```python
from build123d import *

# Parameters (mm, degrees)
CROQUIS1_R              = 1.2
SALIENTE_EXTRUIR1_DEPTH = 1.6
CROQUIS2_W              = 15.7
CROQUIS2_H              = 12.8
SALIENTE_EXTRUIR2_DEPTH = 16


with BuildPart() as part:
    # Croquis1 → Saliente-Extruir1 (new body)
    with BuildSketch(Plane.XY):
        Polygon((55.2, -30.15), (-55.2, -30.15), (-55.2, 27.15), (-52.2, 30.15), (52.2, 30.15), (55.2, 27.15), align=None)
        with Locations((-51.1, 26.05)):
            Circle(CROQUIS1_R, mode=Mode.SUBTRACT)
        with Locations((51.1, 26.05)):
            Circle(CROQUIS1_R, mode=Mode.SUBTRACT)
    extrude(amount=SALIENTE_EXTRUIR1_DEPTH)

    # Croquis2 → Saliente-Extruir2 (add)
    with BuildSketch(Plane.XY.offset(1.6)):
        with Locations((-19.55, -17.25)):
            Rectangle(CROQUIS2_W, CROQUIS2_H)
        with Locations((-2.95, -17.25)):
            Rectangle(CROQUIS2_W, CROQUIS2_H)
        with Locations((38.95, -17.25)):
            Rectangle(CROQUIS2_W, CROQUIS2_H)
    extrude(amount=SALIENTE_EXTRUIR2_DEPTH)


solid = part.part
```
The model under review builds one solid part; all positions refer to its coordinate system, in mm. A direction names the side the tool comes from. Give positions to 0.01 mm unless a question says otherwise; leave off trailing zeros. Write each loop counter-clockwise with the first axis right and the second up, starting at its lowest first coordinate (ties: lowest second). Pieces come first, ordered by that corner, then holes. Notation, with made-up numbers: M 53.25,-27.5 L 76.25,-27.5 A36 ccw 76.25,11.5 Z; hole C 10,35 d11. An arc over 180 degrees is marked long. Write each question's results on one line, items separated by ' | '. Start each with the question number.
1. We need section C-C (y = 26.05). Write out the cut boundary in (x, z), and give its area (3 significant figures).
2. Insertion check: pin 1 Ø4 at (y, z) = (-15, 12.5) entering from -X; pin 2 Ø5 at (y, z) = (-23, 5) entering from +X; pin 3 Ø1.5 at (x, z) = (42.5, 14) entering from +Y. Each pin has a flat end and moves straight along its axis. Give the tip position at first contact, or say it passes through.
3. We need section A-A (x = 51.1). Write out the cut boundary in (y, z), and give its area (3 significant figures).
4. We need section D-D (x = -18). Write out the cut boundary in (y, z), and give its area (3 significant figures).
5. For probe 1 along X at (y, z) = (-11, 2); probe 2 along Y at (x, z) = (51.1, 1); probe 3 along Y at (x, z) = (33, 2), list the stretches that pass through material, from the lowest coordinate up. Write a range as [from, to].
6. Mouldability with a two-part tool opening along X and no side actions: class faces 1 (the flat face through (-3, -23.65, 9)), 2 (the flat face through (-11.7, -17, 9)), 3 (the flat face through (46.8, -17, 9)) as released by +X, released by -X, zero draft, split by the parting line, or undercut.
7. For faces 4 (the flat face through (39, -10.85, 9)), 5 (the flat face through (4.9, -17, 9)), 6 (the flat face through (-27.4, -17, 9)), 7 (the flat face through (-20, -23.65, 9)), list the 3-axis set-ups (+Z, -Z, +X, -X, +Y, -Y) from which the entire face can be reached by the end or side of a thin tool; tool diameter is ignored.
8. We need section B-B (z = 15.25). Write out the cut boundary in (x, y), and give its area (3 significant figures).
Results found:
1) outline: M -55.2,0 L -52.3,0 L -52.3,1.6 L -55.2,1.6 Z; M -49.9,0 L 49.9,0 L 49.9,1.6 L -49.9,1.6 Z; M 52.3,0 L 55.2,0 L 55.2,1.6 L 52.3,1.6 Z | area: 169 mm^2
2) pin 1: stops at x = -27.4 | pin 2: stops at x = 46.8 | pin 3: stops at y = -10.85
3) outline: M -30.15,0 L 24.85,0 L 24.85,1.6 L -30.15,1.6 Z; M 27.25,0 L 30.15,0 L 30.15,1.6 L 27.25,1.6 Z | area: 92.6 mm^2
4) outline: M -30.15,0 L 30.15,0 L 30.15,1.6 L -10.85,1.6 L -10.85,17.6 L -23.65,17.6 L -23.65,1.6 L -30.15,1.6 Z | area: 301 mm^2
5) probe 1: x = [-27.4, -11.7], [-10.8, 4.9], [31.1, 46.8] | probe 2: y = [-30.15, 24.85], [27.25, 30.15] | probe 3: y = [-23.65, -10.85]
6) face 1: zero draft | face 2: undercut | face 3: released by +X
7) face 4: +Z, +X, -X, +Y | face 5: +Z, +Y, -Y | face 6: +Z, -X, +Y, -Y | face 7: +Z, +X, -X, -Y
8) outline: M -27.4,-23.65 L -11.7,-23.65 L -11.7,-10.85 L -27.4,-10.85 Z; M -10.8,-23.65 L 4.9,-23.65 L 4.9,-10.85 L -10.8,-10.85 Z; M 31.1,-23.65 L 46.8,-23.65 L 46.8,-10.85 L 31.1,-10.85 Z | area: 603 mm^2
